```python
from build123d import *

# Parameters (mm, degrees)
BOSS_EXTRUDE1_DEPTH = 20
SKETCH2_W           = 0.8000000000000007
SKETCH2_H           = 0.7999999999999989
SKETCH2_H_2         = 0.8000000000000007
CHAMFER1_SIZE       = 0.4
FILLET2_R           = 2
SKETCH3_R           = 2.100000000000004
SKETCH3_R_2         = 2.100000000000001
CUT_EXTRUDE1_DEPTH  = 44.67007193971907


# Some blends are built 0.0001 mm under size
with BuildPart() as part:
    # Sketch1 → Boss-Extrude1 (new body)
    with BuildSketch(Plane.XY):
        with BuildLine():
            Line((0.9198479389646088, 14.89190109356241), (0.9198479389646088, 2.89190109356241))
            Line((0.9198479389646081, 2.89190109356241), (8.919847938964608, 2.89190109356241))
            ThreePointArc((8.919847938964608, 2.8919010935624105), (10.919847938964608, 4.89190109356241), (12.919847938964608, 2.89190109356241))
            Line((12.919847938964608, 2.89190109356241), (13.669847938964606, 2.89190109356241))
            ThreePointArc((13.669847938964608, 2.8919010935624114), (18.919847938964608, 8.14190109356241), (24.169847938964608, 2.89190109356241))
            Line((24.169847938964608, 2.89190109356241), (24.919847938964608, 2.89190109356241))
            ThreePointArc((24.919847938964608, 2.8919010935624105), (26.919847938964608, 4.891901093562406), (28.919847938964608, 2.89190109356241))
            Line((28.919847938964605, 2.89190109356241), (36.91984793896461, 2.89190109356241))
            Line((36.91984793896461, 2.89190109356241), (36.91984793896461, 14.89190109356241))
            Line((36.91984793896461, 14.89190109356241), (0.9198479389646088, 14.89190109356241))
        make_face()
    extrude(amount=BOSS_EXTRUDE1_DEPTH)

    # Sweep2: sweep along a curve in space
    with BuildLine() as sweep2_path:
        ThreePointArc((24.169847938964608, 2.89190109356241, 20), (22.632158540193984, 6.604211694791784, 20), (18.919847938964608, 8.141901093562412, 20))
        ThreePointArc((18.919847938964608, 8.141901093562412, 20), (15.207537337735232, 6.604211694791786, 20), (13.669847938964606, 2.89190109356241, 20))
    # Sketch2 → Sweep2 (sweep)
    with BuildSketch(Plane.XZ.offset(-2.89190109356241)):
        with Locations((14.069847938964607, 13.400000000000006)):
            Rectangle(SKETCH2_W, SKETCH2_H)
        with Locations((14.069847938964607, 10.400000000000004)):
            Rectangle(SKETCH2_W, SKETCH2_H_2)
        with Locations((14.069847938964607, 7.400000000000003)):
            Rectangle(SKETCH2_W, SKETCH2_H_2)
        Polygon((13.669847938964608, 4.8000000000000025), (14.469847938964607, 4.8000000000000025), (14.469847938964609, 4.000000000000002), (13.669847938964608, 4.000000000000002), align=None)
    sweep(path=sweep2_path.line)

    # Chamfer1
    chamfer1_edges = [part.edges().sort_by_distance(p)[0] for p in [
        (18.919847938964608, 7.341901093562408, 4.000000000000002),
        (18.919847938964608, 7.341901093562411, 4.8000000000000025),
        (18.919847938964608, 7.341901093562411, 7.0000000000000036),
        (18.919847938964608, 7.341901093562413, 7.800000000000004),
        (18.919847938964608, 7.341901093562413, 13.800000000000004),
        (18.919847938964608, 7.341901093562411, 13.000000000000005),
        (18.919847938964608, 7.341901093562413, 10.800000000000004),
        (18.919847938964608, 7.341901093562411, 10.000000000000004),
    ]]
    chamfer(chamfer1_edges, length=CHAMFER1_SIZE - 0.0001)  # a hair under: the kernel refuses the full size

    # Fillet2
    # the kernel refuses this fillet: 2 mm, written as the material it takes off along each edge
    with BuildSketch(Plane(origin=(10.919847938964608, 2.89190109356241, 0), x_dir=(-0.003141587485879782, -0.9999950652018582, 0), z_dir=(0.9999950652018582, -0.003141587485879782, 0))) as fillet2_piece_1:
        with BuildLine():
            CenterArc((2 + FILLET2_R, -FILLET2_R), FILLET2_R, 89.99999999999997, 90)
            Line((2 + FILLET2_R, 2.2e-16), (2, 0))
            Line((2, 0), (2, -FILLET2_R))
        make_face()
    revolve(axis=Axis((10.919847938964608, 2.89190109356241, 0), (0, 0, -1)), revolution_arc=359.64000000000004, mode=Mode.SUBTRACT)
    with BuildSketch(Plane(origin=(26.919847938964608, 2.8919010935624057, 0), x_dir=(-0.003141587485879782, -0.9999950652018582, 0), z_dir=(0.9999950652018582, -0.003141587485879782, 0))) as fillet2_piece_2:
        with BuildLine():
            CenterArc((2.000000000000005 + FILLET2_R, -FILLET2_R), FILLET2_R, 90, 90)
            Line((2.000000000000005, -FILLET2_R), (2.000000000000005, 0))
            Line((2.000000000000005, 0), (2.000000000000005 + FILLET2_R, 0))
        make_face()
    revolve(axis=Axis((26.919847938964608, 2.8919010935624057, 0), (0, 0, -1)), revolution_arc=359.64, mode=Mode.SUBTRACT)
    with BuildSketch(Plane(origin=(10.919847938964608, 2.89190109356241, 20), x_dir=(-0.003141587485879782, -0.9999950652018582, 0), z_dir=(0.9999950652018582, -0.003141587485879782, 0))) as fillet2_piece_3:
        with BuildLine():
            CenterArc((2.0000000000000058 + FILLET2_R, FILLET2_R), FILLET2_R, 180, 90)
            Line((2.0000000000000058, FILLET2_R), (2.0000000000000058, 0))
            Line((2.0000000000000058, 0), (2.0000000000000058 + FILLET2_R, 0))
        make_face()
    revolve(axis=Axis((10.919847938964608, 2.89190109356241, 20), (0, 0, -1)), revolution_arc=359.64000000000004, mode=Mode.SUBTRACT)
    with BuildSketch(Plane(origin=(26.919847938964608, 2.8919010935624057, 20), x_dir=(-0.003141587485879782, -0.9999950652018582, 0), z_dir=(0.9999950652018582, -0.003141587485879782, 0))) as fillet2_piece_4:
        with BuildLine():
            CenterArc((2.000000000000005 + FILLET2_R, FILLET2_R), FILLET2_R, 180, 90)
            Line((2.000000000000005, FILLET2_R), (2.000000000000005, 0))
            Line((2.000000000000005, 0), (2.000000000000005 + FILLET2_R, 0))
        make_face()
    revolve(axis=Axis((26.919847938964608, 2.8919010935624057, 20), (0, 0, -1)), revolution_arc=359.64, mode=Mode.SUBTRACT)

    # Sketch3 → Cut-Extrude1 (cut, through all)
    with BuildSketch(Plane.XZ.offset(-2.89190109356241)):
        with Locations(Location((32.9198479389646, 10, 0), (0, 0, 270))):
            Circle(SKETCH3_R)
        with Locations(Location((4.919847938964609, 10, 0), (0, 0, 270))):
            Circle(SKETCH3_R_2)
    extrude(amount=-CUT_EXTRUDE1_DEPTH, mode=Mode.SUBTRACT)


solid = part.part
```
For this review, take the finished solid that the model builds, in its own axes (mm). A direction names the side the tool comes from. Round coordinates to 2 decimals unless told otherwise and drop trailing zeros. Write each loop counter-clockwise with the first axis right and the second up, starting at its lowest first coordinate (ties: lowest second). Pieces come first, ordered by that corner, then holes. Notation, with made-up numbers: M -20,37 L -14,37 A25 ccw -14,64 Z; hole C -18,84.5 d5. An arc over 180 degrees is marked long. One line per item, written item: value. Start each with the question number.
(1) The part is to be moulded in two halves that separate along X. For faces 1 (the flat face through (36.92, 9, 10)), 2 (the flat face through (4.9, 2.892, 7.6)), 3 (the cylindrical face through (10.88, 4.89, 9.89)), say which applies: released by +X, released by -X, zero draft, split by the parting line, or undercut.
(2) We need section B-B (x = 6.5). Give the boundary of the cut face in (y, z), and give its area (3 significant figures).
(3) We need section D-D (y = 4.5). Count the separate pieces of the cut face and the enclosed holes in it, and give its area (3 significant figures).
(4) We need section A-A (z = 5.5). Give the boundary of the cut face in (x, y).
(5) We need section C-C (y = 10). Give the boundary of the cut face in (x, z), and give its area (3 significant figures).
(6) Wall thickness on line 1 (X direction, y = 9, z = 10); line 2 (X direction, y = 3.75, z = 10.25); line 3 (X direction, y = 4.25, z = 1.75): over which ranges is each line inside the solid? List them lowest first.
(7) Insertion check: pin 1 (2.5 mm diameter, centred on x = 21, y = 6, fed in from +Z); pin 2 (1.5 mm diameter, centred on x = 11, z = 2.5, fed in from -Y); pin 3 (2.5 mm diameter, centred on x = 21.5, y = 5.5, fed in from -Z). Each pin has a flat end and moves straight along its axis. Give the tip position at first contact, or say it passes through.
(8) Machinability: for faces 4 (the cylindrical face through (26.88, 4.89, 9.89)), 5 (the conical face through (19.02, 7.45, 7.51)), 6 (the cylindrical face through (18.8, 8.14, 1.97)), which of the approach directions +Z, -Z, +X, -X, +Y, -Y give a long, thin tool a straight path to every point of the face, cutting with its end or side? Answer none if there is none.
Result:
1. face 1: released by +X
1. face 2: zero draft
1. face 3: undercut
2. outline: M 2.89,0 L 14.89,0 L 14.89,8.62 L 2.89,8.62 Z; M 2.89,11.38 L 14.89,11.38 L 14.89,20 L 2.89,20 Z
2. area: 207 mm²
3. separate pieces: 4
3. enclosed holes: 2
3. area: 392 mm²
4. outline: M 0.92,2.89 L 8.92,2.89 A2 cw 12.92,2.89 L 13.67,2.89 A5.25 cw 24.17,2.89 L 24.92,2.89 A2 cw 28.92,2.89 L 36.92,2.89 L 36.92,14.89 L 0.92,14.89 Z
5. outline: M 0.92,0 L 36.92,0 L 36.92,20 L 0.92,20 Z; hole C 4.92,10 d4.2; hole C 32.92,10 d4.2
5. area: 692 mm²
6. line 1: 0.92 to 2.82, 7.02 to 30.82, 35.02 to 36.92
6. line 2: 0.92 to 2.83, 7 to 9.11, 12.73 to 14.4, 23.44 to 25.11, 28.73 to 30.83, 35 to 36.92
6. line 3: 0.92 to 9.43, 12.41 to 13.85, 23.99 to 25.43, 28.41 to 36.92
7. pin 1: z = 13.8
7. pin 2: y = 4.71
7. pin 3: z = 4
8. face 4: +Z, -Z, -Y
8. face 5: -Y
8. face 6: -Z, -Y
